```python
from build123d import *

# Parameters (mm, degrees)
SKETCH_1_W          = 52.9
SKETCH_1_H          = 77
EXTRUDE_1_DEPTH     = 2
SKETCH_1_3_W        = 0.8
SKETCH_1_3_H        = 77
EXTRUDE_2_DEPTH     = 0.8
SKETCH_2_W          = 54.5
SKETCH_2_H          = 0.9
EXTRUDE_3_DEPTH     = 0.8
SKETCH_3_W          = 4.8
SKETCH_3_H          = 0.9
CUT_EXTRUDE_1_DEPTH = 0.8
EXTRUDE_START       = -38.5
EXTRUDE_4_DEPTH     = 77


with BuildPart() as part:
    # 草图1 → 凸台-拉伸1 (new body)
    with BuildSketch(Plane(origin=(0, 0, 0), x_dir=(1, 0, 0), z_dir=(0, 1, 0))):
        Rectangle(SKETCH_1_W, SKETCH_1_H)
    extrude(amount=EXTRUDE_1_DEPTH)

    # 草图1<3> → 凸台-拉伸2 (add)
    with BuildSketch(Plane(origin=(0, 0, 0), x_dir=(1, 0, 0), z_dir=(0, 1, 0))):
        with Locations((26.85, 0)):
            Rectangle(SKETCH_1_3_W, SKETCH_1_3_H)
        with Locations((-26.85, 0)):
            Rectangle(SKETCH_1_3_W, SKETCH_1_3_H)
    extrude(amount=EXTRUDE_2_DEPTH)

    # 草图2 → 凸台-拉伸3 (add)
    with BuildSketch(Plane(origin=(0, 0, 0), x_dir=(1, 0, 0), z_dir=(0, 1, 0))):
        with Locations((0, -38.95)):
            Rectangle(SKETCH_2_W, SKETCH_2_H)
    extrude(amount=EXTRUDE_3_DEPTH)

    # 草图3 → 切除-拉伸1 (cut)
    with BuildSketch(Plane(origin=(0, 0, 0), x_dir=(1, 0, 0), z_dir=(0, 1, 0))):
        with Locations((-24.85, -38.95)):
            Rectangle(SKETCH_3_W, SKETCH_3_H)
        with Locations((24.85, -38.95)):
            Rectangle(SKETCH_3_W, SKETCH_3_H)
    extrude(amount=CUT_EXTRUDE_1_DEPTH, mode=Mode.SUBTRACT)

    # 草图4 → 凸台-拉伸4 (add)
    with BuildSketch(Plane.XY.offset(EXTRUDE_START)):
        Polygon((22.45, 3), (22.45, 5), (32.95, 5), (32.95, 0), (30.95, 0), (30.95, 3), (26.45, 3), (26.45, 2), (22.45, 2), align=None)
        Polygon((-30.95, 0), (-30.95, 3), (-26.45, 3), (-26.45, 2), (-22.45, 2), (-22.45, 3), (-22.45, 5), (-32.95, 5), (-32.95, 0), align=None)
    extrude(amount=EXTRUDE_4_DEPTH)


solid = part.part
```
Part model, mm, in its own coordinate system. A direction names the side the tool comes from. Give positions to 0.01 mm unless a question says otherwise; leave off trailing zeros. Write each loop counter-clockwise with the first axis right and the second up, starting at its lowest first coordinate (ties: lowest second). Pieces come first, ordered by that corner, then holes. Notation, with made-up numbers: (-9, 0) -> (38, 0) arc R20 cw to (38, 38) -> close; hole circle Ø6 at (49, 77.5). An arc over 180 degrees is marked (long way). Put each result on its own line as item: value. Start each with the question number.
Item 1: Cut at A-A (x = -11.5). List the corners of the cut face in (y, z), then the cut area to 3 significant figures.
Item 2: Pull direction X, two halves, no side cores. Call faces 1 (the face through (-26.45, 2, 1)), 2 (the face through (32.95, 3, -1)), 3 (the face through (-28, 5, -1)), 4 (the face through (-32.95, 3, -1)): pulls with the +X half, pulls with the -X half, needs draft (parallel to the pull), parting line crosses it, or undercut.
Item 3: Pin check, flat tips, straight feed: pin 1 Ø0.6 at (y, z) = (0.5, 39) entering from -X; pin 2 Ø22.5 at (x, z) = (6, -7) entering from +Y; pin 3 Ø1.3 at (x, z) = (-29.5, 15.5) entering from -Y. Stop position of each tip, or through.
Item 4: Cut at B-B (z = 31). List the corners of the cut face in (x, y).
Item 5: Which spindle directions (+Z, -Z, +X, -X, +Y, -Y) get a long thin tool onto all of the face, cutting with end or side? Do faces 5 (the face through (-29, 3, -1)), 6 (the face through (0, 2, -1)), 7 (the face through (-30.95, 1, -1)). Say none if no direction does.
Item 6: Wall check: L1, parallel to X at y = 2.8, z = -31; L2, parallel to X at y = 1.05, z = 2.5; L3, parallel to X at y = 0.5, z = -34.5. Give the ranges that are in metal, low to high. Write a range as [from, to].
Answer list:
1. outline: (0, -38.5) -> (2, -38.5) -> (2, 38.5) -> (0.8, 38.5) -> (0.8, 39.4) -> (0, 39.4) -> close
1. area: 155 mm2
2. face 1: undercut
2. face 2: pulls with the +X half
2. face 3: needs draft
2. face 4: pulls with the -X half
3. pin 1: stops at x = -22.45
3. pin 2: stops at y = 2
3. pin 3: stops at y = 3
4. outline: (-32.95, 0) -> (-30.95, 0) -> (-30.95, 3) -> (-26.45, 3) -> (-26.45, 0.8) -> (-27.25, 0.8) -> (-27.25, 0) -> (27.25, 0) -> (27.25, 0.8) -> (26.45, 0.8) -> (26.45, 3) -> (30.95, 3) -> (30.95, 0) -> (32.95, 0) -> (32.95, 5) -> (22.45, 5) -> (22.45, 2) -> (-22.45, 2) -> (-22.45, 5) -> (-32.95, 5) -> close
5. face 5: +Z, -Z
5. face 6: +Z, -Z, +Y
5. face 7: +Z, -Z, -Y
6. L1: x = [-32.95, -30.95], [-26.45, -22.45], [22.45, 26.45], [30.95, 32.95]
6. L2: x = [-32.95, -30.95], [-26.45, 26.45], [30.95, 32.95]
6. L3: x = [-32.95, -30.95], [-27.25, 27.25], [30.95, 32.95]
